Input: part model. Units: mm. Frame: model coordinates. A direction names the side the tool comes from. Round coordinates to 2 decimals unless told otherwise and drop trailing zeros. Write each loop counter-clockwise with the first axis right and the second up, starting at its lowest first coordinate (ties: lowest second). Pieces come first, ordered by that corner, then holes. Notation, with made-up numbers: M 73.5,7.5 L 132.5,7.5 A32 ccw 132.5,45.5 Z; hole C 86,57.25 d10. An arc over 180 degrees is marked long. Answer as CSV lines item,"result". Start each with the question number.
```python
from build123d import *

# Parameters (mm, degrees)
SKETCH2_W           = 12
SKETCH2_H           = 60
BOSS_EXTRUDE1_DEPTH = 12.5
SKETCH3_W           = 8
SKETCH3_H           = 12.5
CUT_EXTRUDE1_DEPTH  = 35.644624403
SKETCH4_R           = 2.25
CUT_EXTRUDE2_DEPTH  = 36
FILLET1_R           = 5
FILLET2_R           = 4
CUT_EXTRUDE3_START  = -8
SKETCH5_R           = 5
CUT_EXTRUDE3_DEPTH  = 4
SKETCH6_R           = 7.5
CUT_EXTRUDE4_DEPTH  = 4
SKETCH8_R           = 5.5
CUT_EXTRUDE6_DEPTH  = 5


with BuildPart() as part:
    # Sketch2 → Boss-Extrude1 (new, symmetric)
    with BuildSketch(Plane.XY):
        Rectangle(SKETCH2_W, SKETCH2_H)
    extrude(amount=BOSS_EXTRUDE1_DEPTH, both=True)

    # Sketch3 → Cut-Extrude1 (cut, through all)
    with BuildSketch(Plane(origin=(6, 0, 0), x_dir=(0, 0, -1), z_dir=(1, 0, 0))):
        with Locations((-8.5, -23.75)):
            Rectangle(SKETCH3_W, SKETCH3_H)
        with Locations((8.5, -23.75)):
            Rectangle(SKETCH3_W, SKETCH3_H)
        with Locations((8.5, 23.75)):
            Rectangle(SKETCH3_W, SKETCH3_H)
        with Locations((-8.5, 23.75)):
            Rectangle(SKETCH3_W, SKETCH3_H)
    extrude(amount=-CUT_EXTRUDE1_DEPTH, mode=Mode.SUBTRACT)

    # Sketch4 → Cut-Extrude2 (cut, through all)
    with BuildSketch(Plane.XY.offset(4.5)):
        with Locations((-1, 25)):
            Circle(SKETCH4_R)
        with Locations((-1, -24.5)):
            Circle(SKETCH4_R)
    extrude(amount=-CUT_EXTRUDE2_DEPTH, mode=Mode.SUBTRACT)

    # Fillet1
    fillet1_edges = [part.edges().sort_by_distance(p)[0] for p in [
        (0, 17.5, 12.5),
        (0, 17.5, -12.5),
        (0, -17.5, -12.5),
        (0, -17.5, 12.5),
    ]]
    fillet(fillet1_edges, radius=FILLET1_R)

    # Fillet2
    fillet2_edges = [part.edges().sort_by_distance(p)[0] for p in [
        (6, -30, 0),
        (-6, -30, 0),
        (-6, 30, 0),
        (6, 30, 0),
    ]]
    fillet(fillet2_edges, radius=FILLET2_R)

    # Sketch5 → Cut-Extrude3 (cut)
    with BuildSketch(Plane.ZY.offset(6).offset(CUT_EXTRUDE3_START)):
        with Locations(Location((0, 0, 0), (0, 0, 270))):
            Circle(SKETCH5_R)
    extrude(amount=-CUT_EXTRUDE3_DEPTH, mode=Mode.SUBTRACT)

    # Sketch6 → Cut-Extrude4 (cut)
    with BuildSketch(Plane.ZY.offset(6)):
        with Locations(Location((0, 0, 0), (0, 0, 270))):
            Circle(SKETCH6_R)
    extrude(amount=-CUT_EXTRUDE4_DEPTH, mode=Mode.SUBTRACT)

    # Sketch8 → Cut-Extrude6 (cut)
    with BuildSketch(Plane.ZY.offset(2)):
        with Locations(Location((0, 0, 0), (0, 0, 270))):
            Circle(SKETCH8_R)
    extrude(amount=-CUT_EXTRUDE6_DEPTH, mode=Mode.SUBTRACT)


solid = part.part
```
Item 1: Draft query along Z for faces 1 (the face through (0, -30, 0)), 2 (the face through (-0.08, 16.07, -11)), 3 (the face through (0.46, 1.19, -5.37)). Return one class per face: +Z half, -Z half, draft (parallel to the pull), parting line (faces both ways), or undercut.
Item 2: Cut plane C-C, the plane z = 0. Return loops of the section in (x, y).
Item 3: Cut plane A-A, the plane x = -1. Return loops of the section in (y, z).
Item 4: Cut plane D-D, the plane y = 0. Return loops of the section in (x, z).
Item 5: Pin query (flat end, axial travel): pin 1 Ø3.5 at (x, y) = (-0.5, -24) entering from +Z; pin 2 Ø0.9 at (x, z) = (-1, -6.5) entering from -Y; pin 3 Ø6 at (x, y) = (0.5, 26) entering from -Z; pin 4 Ø2.5 at (x, y) = (-1, -24.5) entering from -Z. Return the tip coordinate at first contact, or that it passes through.
Item 6: Cut plane B-B, the plane y = 25. Return loops of the section in (x, z), plus the area to 3 significant figures.
Item 7: Access query for faces 4 (the face through (0, -17.5, 6)), 5 (the face through (0, -17.5, -6)), 6 (the face through (0, 22, 4.5)). Directions: +Z, -Z, +X, -X, +Y, -Y. A direction counts if a zero-diameter tool reaches every point of the face in a straight line with its end or side. Return the directions, or none.
Item 8: Line query: line 1 (Y direction, x = -0.25, z = -4); line 2 (Z direction, x = 1.5, y = 19); line 3 (Z direction, x = 1.25, y = -0.5). Output: solid intervals per line, ascending. Write a range as [from, to].
Results list:
1,face 1,"draft"
1,face 2,"-Z half"
1,face 3,"undercut"
2,outline,"M -6,-26 A4 ccw -2,-30 L 2,-30 A4 ccw 6,-26 L 6,-5 L 3,-5 L 3,-5.5 L -2,-5.5 L -2,-7.5 L -6,-7.5 Z; M -6,7.5 L -2,7.5 L -2,5.5 L 3,5.5 L 3,5 L 6,5 L 6,26 A4 ccw 2,30 L -2,30 A4 ccw -6,26 Z; hole C -1,-24.5 d4.5; hole C -1,25 d4.5"
3,outline,"M -30,-4.5 L -26.75,-4.5 L -26.75,4.5 L -30,4.5 Z; M -22.25,-4.5 L -17.5,-4.5 L -17.5,-7.5 A5 ccw -12.5,-12.5 L 12.5,-12.5 A5 ccw 17.5,-7.5 L 17.5,-4.5 L 22.75,-4.5 L 22.75,4.5 L 17.5,4.5 L 17.5,7.5 A5 ccw 12.5,12.5 L -12.5,12.5 A5 ccw -17.5,7.5 L -17.5,4.5 L -22.25,4.5 Z; M 27.25,-4.5 L 30,-4.5 L 30,4.5 L 27.25,4.5 Z; hole C 0,0 d11"
4,outline,"M -6,-12.5 L 6,-12.5 L 6,-5 L 3,-5 L 3,-5.5 L -2,-5.5 L -2,-7.5 L -6,-7.5 Z; M -6,7.5 L -2,7.5 L -2,5.5 L 3,5.5 L 3,5 L 6,5 L 6,12.5 L -6,12.5 Z"
5,pin 1,"z = 4.5"
5,pin 2,"y = -17.5"
5,pin 3,"z = -4.5"
5,pin 4,"through"
6,outline,"M -6,-4.5 L -3.25,-4.5 L -3.25,4.5 L -6,4.5 Z; M 1.25,-4.5 L 6,-4.5 L 6,4.5 L 1.25,4.5 Z"
6,area,"67.5 mm²"
7,face 4,"+Z, +X, -X, -Y"
7,face 5,"-Z, +X, -X, -Y"
7,face 6,"+Z, +X, -X, +Y"
8,line 1,"[-30, -26.62], [-22.38, -3.77], [3.77, 22.88], [27.12, 30]"
8,line 2,"[-4.5, 4.5]"
8,line 3,"[-12.5, -5.48], [5.48, 12.5]"
